Input: dimensioned drawing with shaded views. Units: mm. Origin: part minimum x, y, z. A direction names the side the tool comes from. Round coordinates to 2 decimals unless told otherwise and drop trailing zeros. Order: outer loops, then holes, each group sorted by start corner. A loop starts at its lowest first (then second) coordinate and runs counter-clockwise, first axis right, second up. Notation, with made-up numbers: M -2.75,-22 L 2.25,-22 A35 cw 2.25,12 Z; hole C 34,67.5 d6. An arc over 180 degrees is marked long. Use one line per item in the form item = value. Start each with the question number.
Q1. Reachability of the marked faces 4 and 5 from +Z, -Z, +X, -X, +Y, -Y: full face, straight path, thin tool, end or side. Return the list, or none.
Q2. Section C-C (y = 56.25). Return the cut outline in (x, z) (3 decimals).
Q3. Section D-D (y = 17.5). Return the cut outline in (x, z).
Q4. Section B-B (x = 9.5). Return the cut outline in (y, z) (3 decimals).
Q5. Contact query for flat-ended pins moving along their axis: pin 1 (1.5 mm diameter, centred on y = 52.5, z = 2.5, fed in from -X); pin 2 (1.5 mm diameter, centred on y = 19, z = 2.5, fed in from +X); pin 3 (1 mm diameter, centred on x = 10.5, z = 1, fed in from -Y). Output: stop coordinate, or through.
Q6. Section A-A (z = 2.6). Return the cut outline in (x, y) (3 decimals), plus the area to 3 significant figures.
Q7. Pull-direction query (Y, two-part tool) for the marked faces 1, 2 and 3; classes: pulls with the +Y half, pulls with the -Y half, needs draft (parallel to the pull), parting line crosses it, or undercut.
Q8. Material intervals for probe 1 along Y at (x, z) = (9.5, 2.15) (3 decimals); probe 2 along Y at (x, z) = (7.75, 2.55); probe 3 along X at (y, z) = (26, 4.65), sorted ascending.
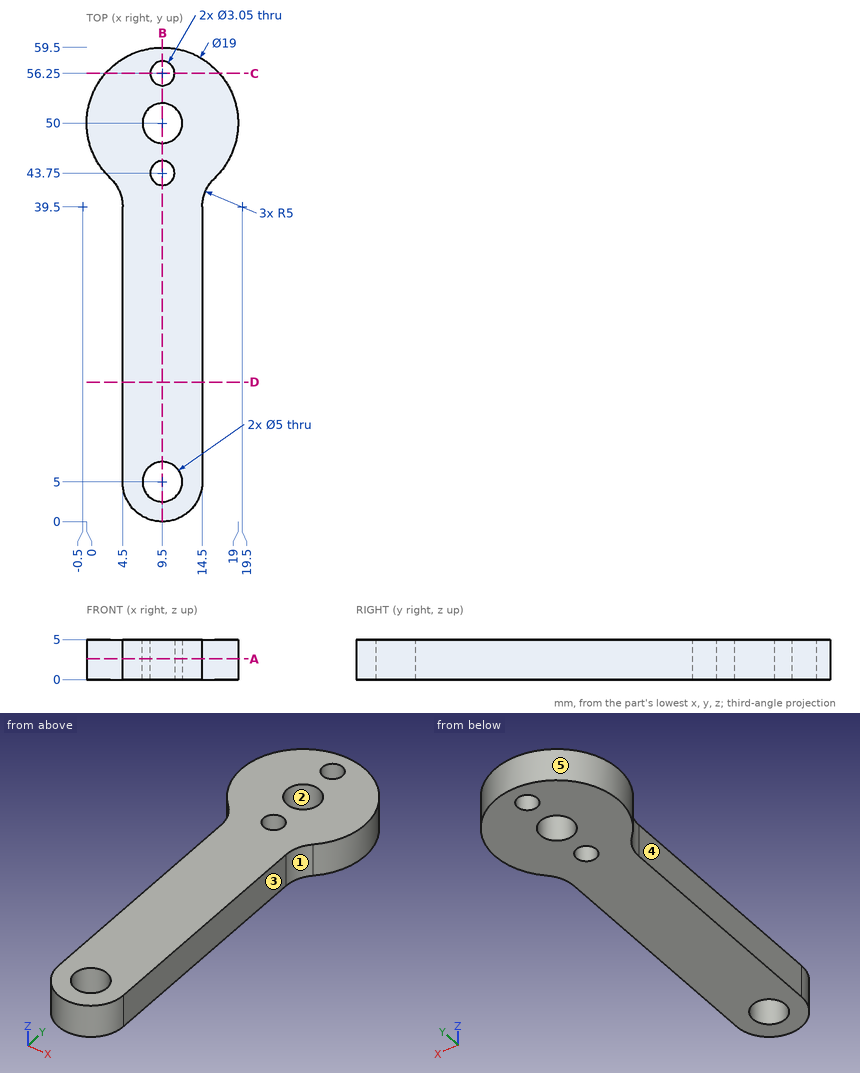
Results list:
q1.face_4 = +Z, -Z, -X, -Y
q1.face_5 = +Z, -Z
q2.outline = M 2.345,0 L 7.975,0 L 7.975,5 L 2.345,5 Z; M 11.025,0 L 16.655,0 L 16.655,5 L 11.025,5 Z
q3.outline = M 4.5,0 L 14.5,0 L 14.5,5 L 4.5,5 Z
q4.outline = M 0,0 L 2.5,0 L 2.5,5 L 0,5 Z; M 7.5,0 L 42.225,0 L 42.225,5 L 7.5,5 Z; M 45.275,0 L 47.5,0 L 47.5,5 L 45.275,5 Z; M 52.5,0 L 54.725,0 L 54.725,5 L 52.5,5 Z; M 57.775,0 L 59.5,0 L 59.5,5 L 57.775,5 Z
q5.pin_1 = 0.16
q5.pin_2 = 14.5
q5.pin_3 = 0.03
q6.outline = M 2.948,43.121 A5 cw 4.5,39.5 L 4.5,5 A5 ccw 14.5,5 L 14.5,39.5 A5 cw 16.052,43.121 A9.5 ccw long Z; hole C 9.5,5 d5; hole C 9.5,50 d5; hole C 9.5,43.75 d3.05; hole C 9.5,56.25 d3.05
q6.area = 630 mm2
q7.face_1 = pulls with the -Y half
q7.face_2 = undercut
q7.face_3 = needs draft
q8.probe_1 = 0 to 2.5, 7.5 to 42.225, 45.275 to 47.5, 52.5 to 54.725, 57.775 to 59.5
q8.probe_2 = 0.32 to 3.21, 6.79 to 48.21, 51.79 to 59.34
q8.probe_3 = 4.5 to 14.5
